Geometry check sheet. Reference: the model listing, model coordinates, mm. A direction names the side the tool comes from. Round coordinates to 2 decimals unless told otherwise and drop trailing zeros. Order: outer loops, then holes, each group sorted by start corner. A loop starts at its lowest first (then second) coordinate and runs counter-clockwise, first axis right, second up.
```python
from build123d import *

# Parameters (mm, degrees)
SKETCH1_W           = 168
SKETCH1_H           = 22
BOSS_EXTRUDE1_DEPTH = 17.8
SKETCH8_R           = 2
CUT_EXTRUDE4_DEPTH  = 22
CUT_EXTRUDE2_REACH  = 88.567
SKETCH5_W           = 117
SKETCH5_H           = 6
CUT_EXTRUDE3_DEPTH  = 15.8
BOSS_EXTRUDE3_REACH = 90.164
SKETCH7_W           = 47
SKETCH7_H           = 2
FILLET1_R           = 7


with BuildPart() as part:
    # Sketch1 → Boss-Extrude1 (new body)
    with BuildSketch(Plane(origin=(0, 0, 0), x_dir=(1, 0, 0), z_dir=(0, 1, 0))):
        Rectangle(SKETCH1_W, SKETCH1_H)
    extrude(amount=-BOSS_EXTRUDE1_DEPTH)

    # Sketch8 → Cut-Extrude4 (cut)
    with BuildSketch(Plane.XY.offset(11)):
        with Locations((79.55, -13.35)):
            Circle(SKETCH8_R)
    extrude(amount=-CUT_EXTRUDE4_DEPTH, mode=Mode.SUBTRACT)

    # Cut-Extrude2: up to this face of the body (flat: up to its plane)
    cut_extrude2_end = Plane(part.part.faces().sort_by_distance((0, -17.8, 0))[0])
    # Sketch5 → Cut-Extrude2 (cut, up to the picked face)
    with BuildSketch(Plane(origin=(0, 0, 0), x_dir=(1, 0, 0), z_dir=(0, 1, 0)), mode=Mode.PRIVATE) as cut_extrude2_sk1:
        with Locations((25.5, 8)):
            Rectangle(SKETCH5_W, SKETCH5_H)
    cut_extrude2_tool1 = split(extrude(cut_extrude2_sk1.sketch, amount=-CUT_EXTRUDE2_REACH, mode=Mode.PRIVATE), bisect_by=cut_extrude2_end, keep=Keep.BOTH, mode=Mode.PRIVATE)
    # Sketch5 → Cut-Extrude2 (cut, up to the picked face)
    with BuildSketch(Plane(origin=(0, 0, 0), x_dir=(1, 0, 0), z_dir=(0, 1, 0)), mode=Mode.PRIVATE) as cut_extrude2_sk2:
        with Locations((25.5, -8)):
            Rectangle(SKETCH5_W, SKETCH5_H)
    cut_extrude2_tool2 = split(extrude(cut_extrude2_sk2.sketch, amount=-CUT_EXTRUDE2_REACH, mode=Mode.PRIVATE), bisect_by=cut_extrude2_end, keep=Keep.BOTH, mode=Mode.PRIVATE)
    add(cut_extrude2_tool1.solids().sort_by(Axis((25.5, 0, -8), (0, -1, 0)))[0], mode=Mode.SUBTRACT)
    add(cut_extrude2_tool2.solids().sort_by(Axis((25.5, 0, 8), (0, -1, 0)))[0], mode=Mode.SUBTRACT)

    # Sketch6 → Cut-Extrude3 (cut)
    with BuildSketch(Plane.XZ.offset(17.8)):
        Polygon((-82, 9), (-82, -9), (-35, -9), (-35, -3), (82, -3), (82, 3), (-35, 3), (-35, 9), align=None)
    extrude(amount=-CUT_EXTRUDE3_DEPTH, mode=Mode.SUBTRACT)

    # Boss-Extrude3: up to this face of the body (flat: up to its plane)
    boss_extrude3_end = Plane(part.part.faces().sort_by_distance((-58.5, -9.9, 9))[0])
    # Sketch7 → Boss-Extrude3 (add, up to the picked face)
    with BuildSketch(Plane.XY.offset(-9), mode=Mode.PRIVATE) as boss_extrude3_sk1:
        with Locations((-58.5, -13.3)):
            Rectangle(SKETCH7_W, SKETCH7_H)
    boss_extrude3_tool1 = split(extrude(boss_extrude3_sk1.sketch, amount=BOSS_EXTRUDE3_REACH, mode=Mode.PRIVATE), bisect_by=boss_extrude3_end, keep=Keep.BOTH, mode=Mode.PRIVATE)
    add(boss_extrude3_tool1.solids().sort_by(Axis((-58.5, -13.3, -9), (0, 0, 1)))[0])

    # Fillet1
    # the kernel refuses this fillet: 7 mm, written as the material it takes off along each edge
    with BuildSketch(Plane(origin=(84, -17.8, 22.5), x_dir=(-1, 0, 0), z_dir=(0, 0, -1))) as fillet1_piece_1:
        with BuildLine():
            CenterArc((FILLET1_R, FILLET1_R), FILLET1_R, 180, 90)
            Line((0, FILLET1_R), (0, 0))
            Line((0, 0), (FILLET1_R, 0))
        make_face()
    extrude(amount=45, mode=Mode.SUBTRACT)


solid = part.part
```
(1) Material ranges on line 1 (Z direction, x = -8, y = -9); line 2 (X direction, y = -8.5, z = -8.75); line 3 (Z direction, x = -59, y = -4), recorded low to high.
Returned:
line 1: z = -5 to -3, 3 to 5
line 2: x = -84 to -82, -35 to -33
line 3: z = -11 to -9, 9 to 11
(2) Sectioned sample at C-C, the plane x = 71. Record the cut outline in (y, z), and give its area (3 significant figures).
Returned:
outline: (-17.8, -5) - (0, -5) - (0, 5) - (-17.8, 5) - (-17.8, 3) - (-2, 3) - (-2, -3) - (-17.8, -3) - close
area: 83.2 mm2
(3) Sectioned sample at B-B, the plane y = -8.5. Record the cut outline in (x, z), and give its area (3 significant figures).
Returned:
outline: (-84, -11) - (-33, -11) - (-33, -5) - (84, -5) - (84, 5) - (-33, 5) - (-33, 11) - (-84, 11) - close; hole (-82, -9) - (-35, -9) - (-35, -3) - (82, -3) - (82, 3) - (-35, 3) - (-35, 9) - (-82, 9) - close
area: 744 mm2
(4) Draft check along Z on faces 5 (the flat face through (-59, -16, -9)), 6 (the cylindrical face through (78.076, -11.998, 4.014)), 7 (the flat face through (-59, -9, 11)), 8 (the flat face through (25, -9, -5)). Enter one of: released by +Z, released by -Z, zero draft, split by the parting line, or undercut.
Returned:
face 5: undercut
face 6: zero draft
face 7: released by +Z
face 8: released by -Z
(5) Depth check by flat-ended pin: P1, Ø5, axis at y = -11, z = 9, coming from the +X side; P2, Ø5, axis at x = 46, z = -6.5, coming from the -Y side; P3, Ø5, axis at x = 79.55, y = -13.35, coming from the +Z side; P4, Ø1.5, axis at x = 32, y = -13, coming from the -Z side. Enter the tip coordinate at first touch or a pass-through.
Returned:
P1: stops at x = -33
P2: stops at y = -17.8
P3: stops at z = 5
P4: stops at z = -5
(6) Sectioned sample at A-A, the plane x = -61. Record the cut outline in (y, z).
Returned:
outline: (-17.8, -11) - (0, -11) - (0, 11) - (-17.8, 11) - (-17.8, 9) - (-14.3, 9) - (-14.3, -9) - (-17.8, -9) - close; hole (-12.3, -9) - (-2, -9) - (-2, 9) - (-12.3, 9) - close
(7) Set-up check for faces 1 (the flat face through (-33, -9, 8)), 2 (the flat face through (-59, -9, -11)), 3 (the flat face through (-35, -7, -6)), 4 (the flat face through (-82, -16, 0)): record each of +Z, -Z, +X, -X, +Y, -Y from which the full face is reachable in a straight line by a thin tool's end or side.
Returned:
face 1: +Z, +X, +Y, -Y
face 2: -Z, +X, -X, +Y, -Y
face 3: none
face 4: -Y
